from build123d import *

# Parameters (mm, degrees)
ESBO_O1_W                  = 20
ESBO_O1_H                  = 40
RESSALTO_EXTRUS_O1_DEPTH   = 15
FURO_ROSCADO_DE_M121_D     = 10.2
FURO_ROSCADO_DE_M122_D     = 10.2
FURO_ROSCADO_DE_M122_DEPTH = 25
FURO_ROSCADO_DE_M122_TIP   = 3.064389157
CHANFRO2_SIZE              = 2


with BuildPart() as part:
    # Esboço1 → Ressalto-extrusão1 (new, symmetric)
    with BuildSketch(Plane(origin=(0, 0, 0), x_dir=(1, 0, 0), z_dir=(0, 1, 0))):
        Rectangle(ESBO_O1_W, ESBO_O1_H)
    extrude(amount=RESSALTO_EXTRUS_O1_DEPTH, both=True)

    # Furo roscado de M121 (through all)
    with Locations(Plane(origin=(0, 15, 0), x_dir=(1, 0, 0), z_dir=(0, 1, 0))):
        with Locations((0, 10)):
            Hole(FURO_ROSCADO_DE_M121_D / 2)

    # Furo roscado de M122
    with Locations(Plane(origin=(0, 15, 0), x_dir=(1, 0, 0), z_dir=(0, 1, 0))):
        with Locations((0, -10)):
            Hole(FURO_ROSCADO_DE_M122_D / 2, depth=FURO_ROSCADO_DE_M122_DEPTH)
            with Locations((0, 0, -(FURO_ROSCADO_DE_M122_DEPTH + FURO_ROSCADO_DE_M122_TIP / 2))):  # 118° drill point
                Cone(0, FURO_ROSCADO_DE_M122_D / 2, FURO_ROSCADO_DE_M122_TIP, mode=Mode.SUBTRACT)

    # Chanfro2
    chanfro2_edges = [part.edges().sort_by_distance(p)[0] for p in [
        (-10, 15, 0),
        (0, 15, 20),
        (10, 15, 0),
        (0, 15, -20),
    ]]
    chamfer(chanfro2_edges, length=CHANFRO2_SIZE)


solid = part.part
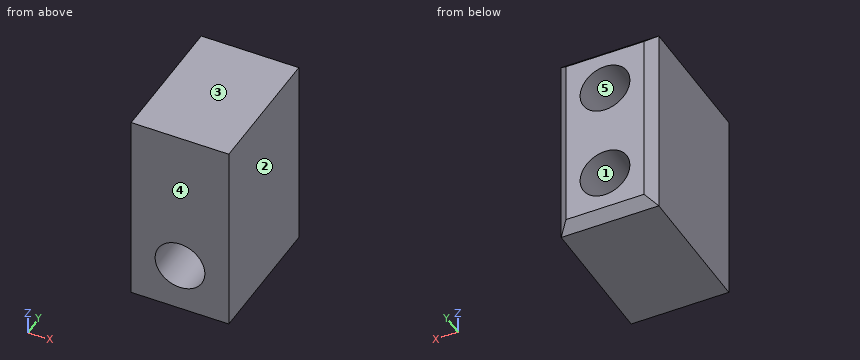
Read the model definition and answer for the solid it produces. Units are mm, in the model's axes. Face numbers are marked on the shaded views. A direction names the side the tool comes from. Round coordinates to 2 decimals unless told otherwise and drop trailing zeros. Write each loop counter-clockwise with the first axis right and the second up, starting at its lowest first coordinate (ties: lowest second). Pieces come first, ordered by that corner, then holes.
Q1. A tool of negligible diameter and unlimited length cuts with its end or side. For the marked faces 4 and 5, from which of +Z, -Z, +X, -X, +Y, -Y can it reach the whole face along a straight path? Write none if from no direction.
Values:
face 4: +Z, -Z, +X, -X, -Y
face 5: +Y
Q2. The mould has two halves that part along X. Classify the marked faces 1, 2 and 3: released by +X, released by -X, zero draft, split by the parting line, or undercut.
Values:
face 1: undercut
face 2: released by +X
face 3: zero draft
Q3. Find section A-A on z = -10. Determine the outline of the cut face in (x, y).
Values:
outline: (-10, -15) - (-5.1, -15) - (-5.1, 15) - (-8, 15) - (-10, 13) - close; (5.1, -15) - (10, -15) - (10, 13) - (8, 15) - (5.1, 15) - close
Q4. A flat-ended cylindrical pin translates along its axis: P1, Ø6, axis at x = 0, z = -10, coming from the -Y side. Find the tip coordinate at first contact, or state that the pin passes through.
Values:
P1: passes through
Q5. Straight lines are drawn through the part: line 1 (Z direction, x = 0, y = 2.25); line 2 (Z direction, x = -1.75, y = 5.25); line 3 (X direction, y = -9.5, z = 6). For each, find the intervals that lie inside material, in ascending order.
Values:
line 1: z = -20 to -15.1, -4.9 to 4.9, 15.1 to 20
line 2: z = -20 to -14.79, -5.21 to 5.21, 14.79 to 20
line 3: x = -10 to -3.16, 3.16 to 10
Q6. Find section C-C on x = -9. Determine the outline of the cut face in (y, z), and give its area (3 significant figures).
Values:
outline: (-15, -20) - (13, -20) - (14, -19) - (14, 19) - (13, 20) - (-15, 20) - close
area: 1,160 mm2
Q7. Find section B-B on y = 9.25. Determine the outline of the cut face in (x, z).
Values:
outline: (-10, -20) - (10, -20) - (10, 20) - (-10, 20) - close; hole circle Ø10.2 at (0, -10); hole circle Ø10.2 at (0, 10)
